Verification items for the finished model (mm, model axes). Face numbers are marked on the shaded views. A direction names the side the tool comes from. Round coordinates to 2 decimals unless told otherwise and drop trailing zeros. Write each loop counter-clockwise with the first axis right and the second up, starting at its lowest first coordinate (ties: lowest second). Pieces come first, ordered by that corner, then holes. Notation, with made-up numbers: (-38, 49.5) - (12, 49.5) arc R11 ccw to (12, 69.5) - close; hole circle Ø1 at (17, 53.5). An arc over 180 degrees is marked (long way). Write each question's results on one line, items separated by ' | '.
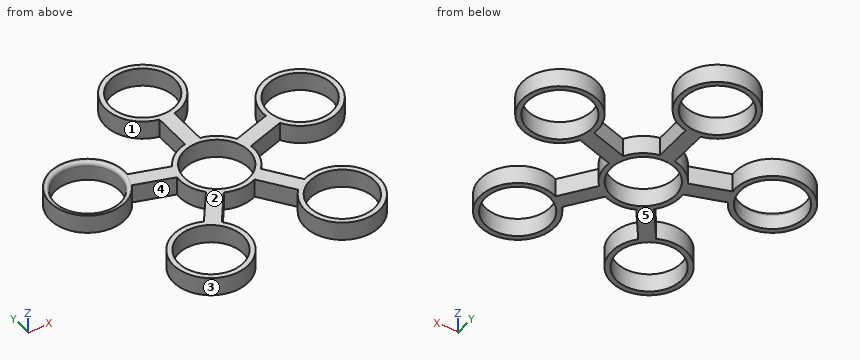
```python
from build123d import *

# Parameters (mm, degrees)
F0_R     = 10.9982
F1_DEPTH = 6.35
F2_R     = 1.27


with BuildPart() as f1:
    # F0 (on Top) → F1 (new body)
    with BuildSketch(Plane.XY):
        with BuildLine():
            Line((-2.54, 25.656592), (-2.54, 12.443408))
            ThreePointArc((-2.54, 12.443408), (-7.464873, 10.274516), (-11.049481, 6.260908))
            Line((-11.049481, 6.260908), (-23.615966, 10.344007))
            ThreePointArc((-23.615966, 10.344007), (-48.313671, 15.698063), (-25.185772, 5.512639))
            Line((-25.185772, 5.512639), (-12.619287, 1.429541))
            ThreePointArc((-12.619287, 1.429541), (-12.078418, -3.924516), (-9.368955, -8.573954))
            Line((-9.368955, -8.573954), (-17.13547, -19.263644))
            ThreePointArc((-17.13547, -19.263644), (-29.859491, -41.098063), (-13.025663, -22.249594))
            Line((-13.025663, -22.249594), (-5.259148, -11.559903))
            ThreePointArc((-5.259148, -11.559903), (0, -12.7), (5.259148, -11.559903))
            Line((5.259148, -11.559903), (13.025663, -22.249594))
            ThreePointArc((13.025663, -22.249594), (29.859491, -41.098063), (17.13547, -19.263644))
            Line((17.13547, -19.263644), (9.368955, -8.573954))
            ThreePointArc((9.368955, -8.573954), (12.078418, -3.924516), (12.619287, 1.429541))
            Line((12.619287, 1.429541), (25.185772, 5.512639))
            ThreePointArc((25.185772, 5.512639), (48.313671, 15.698063), (23.615966, 10.344007))
            Line((23.615966, 10.344007), (11.049481, 6.260908))
            ThreePointArc((11.049481, 6.260908), (7.464873, 10.274516), (2.54, 12.443408))
            Line((2.54, 12.443408), (2.54, 25.656592))
            ThreePointArc((2.54, 25.656592), (0, 50.8), (-2.54, 25.656592))
        make_face()
        with Locations((-22.394618, -30.823547)):
            Circle(F0_R, mode=Mode.SUBTRACT)
        Circle(F0_R, mode=Mode.SUBTRACT)
        with Locations((22.394618, -30.823547)):
            Circle(F0_R, mode=Mode.SUBTRACT)
        with Locations((-36.235253, 11.773547)):
            Circle(F0_R, mode=Mode.SUBTRACT)
        with Locations((0, 38.1)):
            Circle(F0_R, mode=Mode.SUBTRACT)
        with Locations((36.235253, 11.773547)):
            Circle(F0_R, mode=Mode.SUBTRACT)
    extrude(amount=F1_DEPTH)

    # F2
    f2_edges = [f1.edges().sort_by_distance(p)[0] for p in [
        (-47.233453, 11.773547, 6.35),
    ]]
    fillet(f2_edges, radius=F2_R)


solid = f1.part
```
(1) Section check A-A (y = 38.1). Record the cut outline in (x, z), plus the area to 3 significant figures.
Answer:
outline: (-12.7, 0) - (-11, 0) - (-11, 6.35) - (-12.7, 6.35) - close; (11, 0) - (12.7, 0) - (12.7, 6.35) - (11, 6.35) - close | area: 21.6 mm2
(2) Section check C-C (x = 31.5). Record the cut outline in (y, z), plus the area to 3 significant figures.
Answer:
outline: (-39.68, 0) - (-36.99, 0) - (-36.99, 6.35) - (-39.68, 6.35) - close; (-24.65, 0) - (-21.97, 0) - (-21.97, 6.35) - (-24.65, 6.35) - close; (-0.01, 0) - (1.85, 0) - (1.85, 6.35) - (-0.01, 6.35) - close; (21.7, 0) - (23.56, 0) - (23.56, 6.35) - (21.7, 6.35) - close | area: 57.7 mm2
(3) Section check D-D (z = 2.25). Record the cut outline in (x, y), plus the area to 3 significant figures.
Answer:
outline: (-25.19, 5.51) - (-12.62, 1.43) arc R12.7 ccw to (-9.37, -8.57) - (-17.14, -19.26) arc R12.7 ccw (long way) to (-13.03, -22.25) - (-5.26, -11.56) arc R12.7 ccw to (5.26, -11.56) - (13.03, -22.25) arc R12.7 ccw (long way) to (17.14, -19.26) - (9.37, -8.57) arc R12.7 ccw to (12.62, 1.43) - (25.19, 5.51) arc R12.7 ccw (long way) to (23.62, 10.34) - (11.05, 6.26) arc R12.7 ccw to (2.54, 12.44) - (2.54, 25.66) arc R12.7 ccw (long way) to (-2.54, 25.66) - (-2.54, 12.44) arc R12.7 ccw to (-11.05, 6.26) - (-23.62, 10.34) arc R12.7 ccw (long way) to start; hole circle Ø22 at (-36.24, 11.77); hole circle Ø22 at (-22.39, -30.82); hole circle Ø22 at (0, 0); hole circle Ø22 at (0, 38.1); hole circle Ø22 at (22.39, -30.82); hole circle Ø22 at (36.24, 11.77) | area: 1,090 mm2
(4) Mould release check, pull along X, two halves, no side actions. Record for the marked faces 1, 2 and 3: released by +X, released by -X, zero draft, split by the parting line, or undercut.
Answer:
face 1: split by the parting line | face 2: zero draft | face 3: undercut
(5) Set-up check for the marked faces 4 and 5: record each of +Z, -Z, +X, -X, +Y, -Y from which the full face is reachable in a straight line by a thin tool's end or side.
Answer:
face 4: +Z, -Z | face 5: -Z, +X, -X, +Y, -Y
(6) Thickness scan on L1, parallel to Y at x = 0, z = 2.25; L2, parallel to X at y = 20.5, z = 2; L3, parallel to Y at x = -15.5, z = 0.5. Record the ranges inside material, lowest first.
Answer:
L1: -12.7 to -11, 11 to 27.1, 49.1 to 50.8 | L2: -45.46 to -42.93, -29.54 to -27.01, -2.54 to 2.54, 27.01 to 29.54, 42.93 to 45.46 | L3: -41.49 to -39.39, -22.25 to -17.01, 2.37 to 7.71
(7) Go/stop test with flat-tipped pins: pin 1 Ø2 at (x, z) = (21.5, 5) entering from +Y; pin 2 Ø1.5 at (x, z) = (7.5, 4.5) entering from -Y; pin 3 Ø3 at (x, z) = (31, 5.5) entering from -Y. Record where each tip stops, or that it passes through.
Answer:
pin 1: y = 9.98 | pin 2: y = -15.68 | pin 3: y = -41.35
(8) Section check B-B (x = 0). Record the cut outline in (y, z).
Answer:
outline: (-12.7, 0) - (-11, 0) - (-11, 6.35) - (-12.7, 6.35) - close; (11, 0) - (27.1, 0) - (27.1, 6.35) - (11, 6.35) - close; (49.1, 0) - (50.8, 0) - (50.8, 6.35) - (49.1, 6.35) - close
